Verification items for the finished model (mm, model axes). Give positions to 0.01 mm unless a question says otherwise; leave off trailing zeros. Loops run counter-clockwise (first coordinate to the right, second up) from the corner with the lowest first, then second, coordinate; pieces in that order, holes last. Notation, with made-up numbers: M 55.25,74.25 L 105.25,74.25 A23 cw 105.25,109.25 Z; hole C 60,37 d9. An arc over 180 degrees is marked long. Use a Markdown table: item, result.
Autodesk Fusion 360 part; units mm, degrees
sketch "Sketch1" plane through (0, 0, 0) normal (0, 1, 0) x (1, 0, 0)
  circle A0 centre (0, 0) radius 30
  circle A1 centre (0, 0) radius 1
  circle A2 centre (0, 0) radius 2.5
  circle A3 centre (0, 0) radius 28
  dimension "d1" = 60
  dimension "d2" = 2
  dimension "d3" = 5
  dimension "d4" = 56
extrude "Extrude1" add sketch "Sketch1" along normal blind 50 makes body 1 at (29.8509, 16.6667, 2.987) makes body 2 at (2.4876, 16.6667, 0.2489)
sketch "Sketch2" plane through (0, 0, 0) normal (0, 1, 0) x (1, 0, 0)
  line L0 (-13.634, -25.6147) -> (15.366, 24.6147)
  line L1 (15.366, 24.6147) -> (13.634, 25.6147)
  line L2 (13.634, 25.6147) -> (-15.366, -24.6147)
  line L3 (-15.366, -24.6147) -> (-13.634, -25.6147)
  line L4 (-13.634, -25.6147) -> (13.634, 25.6147) construction
  line L5 (15.366, 24.6147) -> (-15.366, -24.6147) construction
  line L6 (13.634, -25.6147) -> (-15.366, 24.6147)
  line L7 (-15.366, 24.6147) -> (-13.634, 25.6147)
  line L8 (-13.634, 25.6147) -> (15.366, -24.6147)
  line L9 (15.366, -24.6147) -> (13.634, -25.6147)
  line L10 (13.634, -25.6147) -> (-13.634, 25.6147) construction
  line L11 (-15.366, 24.6147) -> (15.366, -24.6147) construction
  line L12 (29, 1) -> (-29, 1)
  line L13 (-29, 1) -> (-29, -1)
  line L14 (-29, -1) -> (29, -1)
  line L15 (29, -1) -> (29, 1)
  line L16 (29, 1) -> (-29, -1) construction
  line L17 (-29, 1) -> (29, -1) construction
  dimension "d7" = 58
  dimension "d8" = 2
  dimension "d9" = 58
  dimension "d10" = 2
  dimension "d11" = 58
  dimension "d12" = 2
extrude "Extrude2" add sketch "Sketch2" along normal blind 50 contours L0 L2 L3 L6 L14 | L0 L6 L8 L9 L14 | L2 L6 L12 L13 L14 | L0 L8 L12 L14 L15 | L0 L1 L2 L8 L12 | L2 L6 L7 L8 L12 bodies 1 2
(1) Draft check along X on faces 1 (the cylindrical face through (24.15, 24.65, -14.17)), 2 (the cylindrical face through (-29.97, 24.65, 1.32)), 3 (the flat face through (0, 0, 2)). Enter one of: +X half, -X half, draft (parallel to the pull), parting line (faces both ways), or undercut.
Results below:
| item | result |
|---|---|
| face 1 | undercut |
| face 2 | parting line |
| face 3 | draft |
(2) Cross-section at A-A on z = 0. Record the cut outline in (x, y), then the cut area to 3 significant figures.
Results below:
| item | result |
|---|---|
| outline | M -30,0 L -1,0 L -1,50 L -30,50 Z; M 1,0 L 30,0 L 30,50 L 1,50 Z |
| area | 2,900 mm^2 |
(3) Cross-section at C-C on y = 7.5. Record the cut outline in (x, z).
Results below:
| item | result |
|---|---|
| outline | C 0,0 d60; hole M -27.98,-1 A28 ccw -14.86,-23.73 L -2.01,-1.48 A2.5 cw -2.29,-1 Z; hole M -27.98,1 L -2.29,1 A2.5 cw -2.01,1.48 L -14.86,23.73 A28 ccw Z; hole M -13.13,-24.73 A28 ccw 13.13,-24.73 L 0.28,-2.48 A2.5 cw -0.28,-2.48 Z; hole M -13.13,24.73 L -0.28,2.48 A2.5 cw 0.28,2.48 L 13.13,24.73 A28 ccw Z; hole C 0,0 d2; hole M 2.01,-1.48 L 14.86,-23.73 A28 ccw 27.98,-1 L 2.29,-1 A2.5 cw Z; hole M 2.01,1.48 A2.5 cw 2.29,1 L 27.98,1 A28 ccw 14.86,23.73 Z |
(4) Cross-section at D-D on z = -16.5. Record the cut outline in (x, y), then the cut area to 3 significant figures.
Results below:
| item | result |
|---|---|
| outline | M -25.05,0 L -22.62,0 L -22.62,50 L -25.05,50 Z; M -10.68,0 L -8.37,0 L -8.37,50 L -10.68,50 Z; M 8.37,0 L 10.68,0 L 10.68,50 L 8.37,50 Z; M 22.62,0 L 25.05,0 L 25.05,50 L 22.62,50 Z |
| area | 474 mm^2 |
(5) Cross-section at B-B on x = 4. Record the cut outline in (y, z).
Results below:
| item | result |
|---|---|
| outline | M 0,-29.73 L 50,-29.73 L 50,-27.71 L 0,-27.71 Z; M 0,-8.93 L 50,-8.93 L 50,-4.93 L 0,-4.93 Z; M 0,-1 L 50,-1 L 50,1 L 0,1 Z; M 0,4.93 L 50,4.93 L 50,8.93 L 0,8.93 Z; M 0,27.71 L 50,27.71 L 50,29.73 L 0,29.73 Z |
(6) Gauge pin test, flat ends, axial feed: P1, Ø1, axis at y = 43, z = 1, coming from the +X side; P2, Ø3, axis at x = 17.5, y = 27, coming from the -Z side; P3, Ø10, axis at y = 30, z = 7.5, coming from the -X side; P4, Ø1.8, axis at x = 0, z = 0, coming from the -Y side. Record the tip position at first contact, or that the pin passes through.
Results below:
| item | result |
|---|---|
| P1 | x = 30 |
| P2 | z = -25.38 |
| P3 | x = -29.9 |
| P4 | through |
(7) Material ranges on line 1 (X direction, y = 12, z = 0); line 2 (X direction, y = 28.5, z = 21); line 3 (X direction, y = 3.5, z = 13.5), recorded low to high.
Results below:
| item | result |
|---|---|
| line 1 | -30 to -1, 1 to 30 |
| line 2 | -21.42 to -18.52, -13.28 to -10.97, 10.97 to 13.28, 18.52 to 21.42 |
| line 3 | -26.79 to -24.53, -8.95 to -6.64, 6.64 to 8.95, 24.53 to 26.79 |
